Design review of the part built by this model. Coordinates are the model's own, in mm. A direction names the side the tool comes from. Round coordinates to 2 decimals unless told otherwise and drop trailing zeros. Loops run counter-clockwise (first coordinate to the right, second up) from the corner with the lowest first, then second, coordinate; pieces in that order, holes last. Notation, with made-up numbers: (56, 31) - (83, 31) arc R9 ccw to (83, 47) - close; hole circle Ø3 at (-9.75, 49.5). An arc over 180 degrees is marked (long way). Return JSON: item names as keys, results as strings. Group by question number.
(1) The part is to be moulded in two halves that separate along X. For faces 1 (the flat face through (26, -2, -49)), 2 (the flat face through (0, -1, -52.5)), 3 (the cylindrical face through (29.5, -1.52, -51.07)), say which applies: pulls with the +X half, pulls with the -X half, needs draft (parallel to the pull), parting line crosses it, or undercut.
(2) Clearance check with flat-ended pins moving along their axes: pin 1 (3 mm diameter, centred on x = -3.5, y = 2, fed in from +Z); pin 2 (3 mm diameter, centred on x = -10, z = 16, fed in from +Y); pin 3 (1.6 mm diameter, centred on x = -26, z = -49, fed in from +Y). State where each tip first meets the part, or that it passes through.
(3) Wall thickness on L1, parallel to X at y = 2.25, z = -28; L2, parallel to Z at x = -14.5, y = 2; L3, parallel to X at y = -1.3, z = -49.5: over which ranges is each line inside the solid? List them lowest first. Write a range as [from, to].
(4) We need section D-D, the plane z = -49.5. Write out the cut boundary in (x, y).
(5) We need section C-C, the plane y = 1.5. Write out the cut boundary in (x, z), and give its area (3 significant figures).
(6) We need section A-A, the plane x = -11.5. Write out the cut boundary in (y, z), and give its area (3 significant figures).
(7) We need section B-B, the plane z = 4. Write out the cut boundary in (x, y).
(8) For faces 4 (the flat face through (0, -1, 52.5)), 5 (the flat face through (0, 2, -46)), 6 (the flat face through (28, 2, 1)), 7 (the flat face through (0, 2, 46)), 8 (the cylindrical face through (29.5, -1.52, 51.07)), list the 3-axis set-ups (+Z, -Z, +X, -X, +Y, -Y) from which the entire face can be reached by the end or side of a thin tool; tool diameter is ignored.
from build123d import *

# Parameters (mm, degrees)
SKETCH_1_W          = 62
SKETCH_1_H          = 92
SKETCH_1_W_2        = 56
SKETCH_1_H_2        = 86
EXTRUDE_1_DEPTH     = 3.5
SKETCH_2_W          = 62
SKETCH_2_H          = 105
EXTRUDE_2_DEPTH     = 3
FILLET_2_R          = 5
SKETCH_3_R          = 1.6
CUT_EXTRUDE_1_DEPTH = 2


with BuildPart() as part:
    # 草图1 → 凸台-拉伸1 (new body)
    with BuildSketch(Plane(origin=(0, 0, 0), x_dir=(1, 0, 0), z_dir=(0, 1, 0))):
        Rectangle(SKETCH_1_W, SKETCH_1_H)
        Rectangle(SKETCH_1_W_2, SKETCH_1_H_2, mode=Mode.SUBTRACT)
    extrude(amount=EXTRUDE_1_DEPTH)

    # 草图2 → 凸台-拉伸2 (add)
    with BuildSketch(Plane.XZ):
        Rectangle(SKETCH_2_W, SKETCH_2_H)
    extrude(amount=EXTRUDE_2_DEPTH)

    # 圆角2
    fillet_2_edges = [part.edges().sort_by_distance(p)[0] for p in [
        (31, -1.5, -52.5),
        (31, -1.5, 52.5),
        (-31, -1.5, 52.5),
        (-31, -1.5, -52.5),
    ]]
    fillet(fillet_2_edges, radius=FILLET_2_R)

    # 草图3 → 切除-拉伸1 (cut)
    with BuildSketch(Plane(origin=(0, 0, 0), x_dir=(1, 0, 0), z_dir=(0, 1, 0))):
        with Locations(Location((-26, 49.5, 0), (0, 0, 270))):
            Circle(SKETCH_3_R)
        with Locations(Location((26, 49.5, 0), (0, 0, 90))):
            Circle(SKETCH_3_R)
        with Locations(Location((26, -49.5, 0), (0, 0, 270))):
            Circle(SKETCH_3_R)
        with Locations(Location((-26, -49.5, 0), (0, 0, 90))):
            Circle(SKETCH_3_R)
    extrude(amount=-CUT_EXTRUDE_1_DEPTH, mode=Mode.SUBTRACT)


solid = part.part
Solutions:
{
 "1": {"face 1": "undercut", "face 2": "needs draft", "face 3": "pulls with the +X half"},
 "2": {"pin 1": "z = 46", "pin 2": "y = 0", "pin 3": "y = -2"},
 "3": {"L1": "[-31, -28], [28, 31]", "L2": "[-46, -43], [43, 46]", "L3": "[-30.58, -27.6], [-24.4, 24.4], [27.6, 30.58]"},
 "4": {"outline": "(-30.58, -3) - (30.58, -3) - (30.58, 0) - (27.6, 0) - (27.6, -2) - (24.4, -2) - (24.4, 0) - (-24.4, 0) - (-24.4, -2) - (-27.6, -2) - (-27.6, 0) - (-30.58, 0) - close"},
 "5": {"outline": "(-31, -46) - (31, -46) - (31, 46) - (-31, 46) - close; hole (-28, -43) - (28, -43) - (28, 43) - (-28, 43) - close", "area": "888 mm^2"},
 "6": {"outline": "(-3, -52.5) - (0, -52.5) - (0, -46) - (3.5, -46) - (3.5, -43) - (0, -43) - (0, 43) - (3.5, 43) - (3.5, 46) - (0, 46) - (0, 52.5) - (-3, 52.5) - close", "area": "336 mm^2"},
 "7": {"outline": "(-31, -3) - (31, -3) - (31, 3.5) - (28, 3.5) - (28, 0) - (-28, 0) - (-28, 3.5) - (-31, 3.5) - close"},
 "8": {"face 4": "+Z, +X, -X, +Y, -Y", "face 5": "-Z, +X, -X, +Y", "face 6": "+Y", "face 7": "+Z, +X, -X, +Y", "face 8": "+Z, +X, +Y, -Y"}
}
